```python
from build123d import *

# Parameters (mm, degrees)
SKETCH228_W          = 8
SKETCH228_H          = 2.5
PAD110_DEPTH         = 2
PAD110_DEPTH_BACK    = 6
SKETCH227_R          = 1.05
POCKET092_DEPTH      = 4.001
POCKET092_DEPTH_BACK = 4.001
PAD111_DEPTH         = 4
FILLET001_R          = 0.4
CHAMFER006_SIZE      = 2


with BuildPart() as part:
    # Sketch228 → Pad110 (new body, two sides)
    with BuildSketch(Plane.XY) as pad110_sk:
        with Locations((0, -0.25)):
            Rectangle(SKETCH228_W, SKETCH228_H)
    extrude(amount=PAD110_DEPTH)
    extrude(pad110_sk.sketch, amount=-PAD110_DEPTH_BACK)

    # Sketch227 → Pocket092 (cut, two sides)
    with BuildSketch(Plane.YZ) as pocket092_sk:
        Circle(SKETCH227_R)
    extrude(amount=-POCKET092_DEPTH, mode=Mode.SUBTRACT)
    extrude(pocket092_sk.sketch, amount=POCKET092_DEPTH_BACK, mode=Mode.SUBTRACT)

    # Sketch229 (on Face2 of Pocket092) → Pad111 (join)
    with BuildSketch(Plane(origin=(0, 0, -6), x_dir=(1, 0, 0), z_dir=(0, 0, -1))):
        with BuildLine():
            ThreePointArc((-5, 9.25), (-6.75, 7.5), (-5, 5.75))
            Line((-5, 5.75), (0, 5.75))
            Line((0, 5.75), (0, 1.5))
            Line((0, 1.5), (-4, 1.5))
            Line((-4, 1.5), (-7.331001, 5.6115))
            ThreePointArc((-5, 10.5), (-7.707905, 8.79122), (-7.331001, 5.6115))
            Line((0, 10.5), (-5, 10.5))
            Line((0, 10.5), (0, 9.25))
            Line((-5, 9.25), (0, 9.25))
        make_face()
    pad111 = extrude(amount=-PAD111_DEPTH)

    # Mirrored009: Pad111 across Sketch229 V_Axis
    add(pad111.mirror(Plane(origin=(0, 0, -6), x_dir=(0, 0, -1), z_dir=(1, 0, 0))))

    # Fillet001
    fillet001_edges = [part.edges().sort_by_distance(p)[0] for p in [
        (0, 1, 0.320156),
        (0, 1, -0.320156),
    ]]
    fillet(fillet001_edges, radius=FILLET001_R)

    # Chamfer006
    chamfer006_edges = [part.edges().sort_by_distance(p)[0] for p in [
        (0, 1, -6),
    ]]
    chamfer(chamfer006_edges, length=CHAMFER006_SIZE)


with BuildPart() as part_1:
    # Body081 placement: moved
    add(part.part.moved(Location((162, 7.5, -13))))


solid = part_1.part
```
Input: part model. Units: mm. Frame: model coordinates. A direction names the side the tool comes from. Give positions to 0.01 mm unless a question says otherwise; leave off trailing zeros. Order: outer loops, then holes, each group sorted by start corner. A loop starts at its lowest first (then second) coordinate and runs counter-clockwise, first axis right, second up. Notation, with made-up numbers: M 87,73.5 L 122,73.5 A24 ccw 122,103.5 Z; hole C 33.25,42 d9. An arc over 180 degrees is marked long. One line per question, with ' | ' between items.
1) Access query for faces 1 (the face through (166, 7, -15)), 2 (the face through (162, 1.75, -17)), 3 (the face through (162, 6, -13)), 4 (the face through (158, 7, -15)). Directions: +Z, -Z, +X, -X, +Y, -Y. A direction counts if a zero-diameter tool reaches every point of the face in a straight line with its end or side. Return the directions, or none.
Filled in:
face 1: +Z, -Z, +X, +Y | face 2: +Z, -Z | face 3: +Z, +X, -X, -Y | face 4: +Z, -Z, -X, +Y
2) Ray query, L1, parallel to X at y = 0, z = -16; L2, parallel to X at y = 7.5, z = -17.75; L3, parallel to Y at x = 162.75, z = -15.5. Return the intervals inside material, ascending.
Filled in:
L1: x = 154 to 155.25, 168.75 to 170 | L2: x = 158 to 166 | L3: y = -3 to -1.75, 1.75 to 8.5
3) Section B-B on z = -16.5. Output: boundary loops of the cut face in (x, y).
Filled in:
outline: M 154.67,1.89 A3 ccw 157,-3 L 167,-3 A3 ccw 169.33,1.89 L 166,6 L 166,8.5 L 158,8.5 L 158,6 Z; hole M 157,-1.75 L 167,-1.75 A1.75 ccw 167,1.75 L 157,1.75 A1.75 ccw Z
4) Draft query along X for faces 5 (the face through (162, -1.75, -17)), 6 (the face through (169.69, -1.33, -17.03)), 7 (the face through (162, 3, -19)). Return one class per face: pulls with the +X half, pulls with the -X half, needs draft (parallel to the pull), parting line crosses it, or undercut.
Filled in:
face 5: undercut | face 6: pulls with the +X half | face 7: needs draft
5) Contact query for flat-ended pins moving along their axis: P1, Ø4, axis at y = -0.5, z = -18, coming from the -X side; P2, Ø1.5, axis at x = 167.5, z = -17.5, coming from the +Y side; P3, Ø4, axis at y = 6.5, z = -12.5, coming from the +X side; P4, Ø1.7, axis at y = 7.5, z = -13, coming from the +X side. Output: stop coordinate, or through.
Filled in:
P1: stops at x = 154 | P2: stops at y = 5.07 | P3: stops at x = 166 | P4: passes through
6) Section A-A on y = 0. Output: boundary loops of the cut face in (x, z).
Filled in:
outline: M 154,-19 L 155.25,-19 L 155.25,-15 L 154,-15 Z; M 168.75,-19 L 170,-19 L 170,-15 L 168.75,-15 Z
7) Section C-C on x = 163. Output: boundary loops of the cut face in (y, z).
Filled in:
outline: M -3,-19 L -1.75,-19 L -1.75,-15 L -3,-15 Z; M 1.75,-19 L 6.5,-19 L 8.5,-17 L 8.5,-14.32 A0.4 ccw 7.93,-13.96 A1.05 cw long 7.93,-12.04 A0.4 ccw 8.5,-11.68 L 8.5,-11 L 6,-11 L 6,-15 L 1.75,-15 Z
8) Section D-D on y = 7.5. Output: boundary loops of the cut face in (x, z), and give its area (3 significant figures).
Filled in:
outline: M 158,-18 L 166,-18 L 166,-14.05 L 158,-14.05 Z; M 158,-11.95 L 166,-11.95 L 166,-11 L 158,-11 Z | area: 39.2 mm2
